The drawing under review shows one solid part. Ordinate dimensions are in mm from its lowest x, y, z. A direction names the side the tool comes from. Coordinates: 2 decimals unless noted, no trailing zeros. Loops run counter-clockwise (first coordinate to the right, second up) from the corner with the lowest first, then second, coordinate; pieces in that order, holes last. Notation, with made-up numbers: (2.5, 50) -> (58.5, 50) arc R27 ccw to (58.5, 69) -> close; hole circle Ø3 at (-39.5, 45.5). An arc over 180 degrees is marked (long way). Use a Markdown table: item, result.
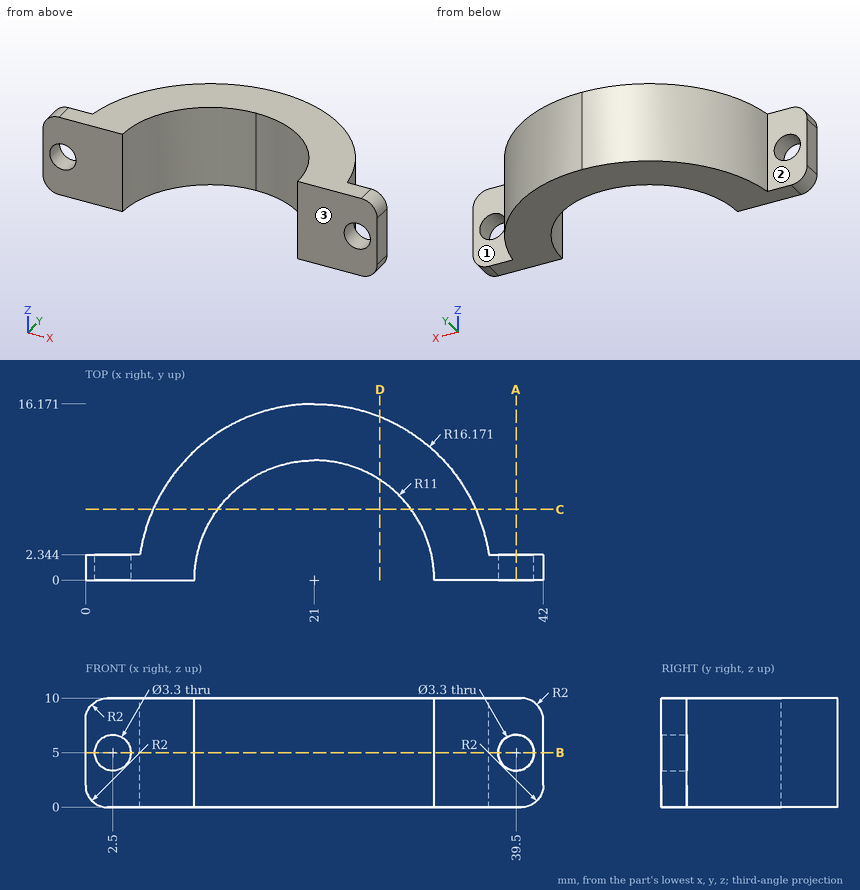
(1) Take a section at C-C on y = 6.5. Write out the cut boundary in (x, z), plus the area to 3 significant figures.
Found:
| item | result |
|---|---|
| outline | (6.19, 0) -> (12.13, 0) -> (12.13, 10) -> (6.19, 10) -> close; (29.87, 0) -> (35.81, 0) -> (35.81, 10) -> (29.87, 10) -> close |
| area | 119 mm^2 |
(2) For pin 1 Ø4 at (x, z) = (18, 2) entering from +Y; pin 2 Ø1.5 at (y, z) = (2.5, 1) entering from +X; pin 3 Ø1.5 at (x, z) = (38.5, 7) entering from +Y, all flat-tipped, find the tip position at first contact; note any pin that passes through.
Found:
| item | result |
|---|---|
| pin 1 | stops at y = 16.14 |
| pin 2 | stops at x = 41.98 |
| pin 3 | stops at y = 2.34 |
(3) For the marked faces 1, 2 and 3, list the 3-axis set-ups (+Z, -Z, +X, -X, +Y, -Y) from which the entire face can be reached by the end or side of a thin tool; tool diameter is ignored.
Found:
| item | result |
|---|---|
| face 1 | +Z, -Z, +X, +Y |
| face 2 | +Z, -Z, -X, +Y |
| face 3 | +Z, -Z, +X, -X, -Y |
(4) Take a section at D-D on x = 27. Write out the cut boundary in (y, z).
Found:
| item | result |
|---|---|
| outline | (9.22, 0) -> (15.02, 0) -> (15.02, 10) -> (9.22, 10) -> close |
(5) Take a section at B-B on z = 5. Write out the cut boundary in (x, y).
Found:
| item | result |
|---|---|
| outline | (0, 0) -> (0.85, 0) -> (0.85, 2.34) -> (0, 2.34) -> close; (4.15, 0) -> (10, 0) arc R11 cw to (32, 0) -> (37.85, 0) -> (37.85, 2.34) -> (37, 2.34) arc R16.17 ccw to (5, 2.34) -> (4.15, 2.34) -> close; (41.15, 0) -> (42, 0) -> (42, 2.34) -> (41.15, 2.34) -> close |
(6) Take a section at A-A on x = 39.5. Write out the cut boundary in (y, z), plus the area to 3 significant figures.
Found:
| item | result |
|---|---|
| outline | (0, 0) -> (2.34, 0) -> (2.34, 3.35) -> (0, 3.35) -> close; (0, 6.65) -> (2.34, 6.65) -> (2.34, 10) -> (0, 10) -> close |
| area | 15.7 mm^2 |
(7) For line 1 along Z through (x, y) = (39.5, 1.3); line 2 along X through (y, z) = (1.75, 5); line 3 along X through (y, z) = (0.9, 5), list the stretches that pass through material, from the lowest coordinate up.
Found:
| item | result |
|---|---|
| line 1 | z = 0 to 3.35, 6.65 to 10 |
| line 2 | x = 0 to 0.85, 4.15 to 10.14, 31.86 to 37.85, 41.15 to 42 |
| line 3 | x = 0 to 0.85, 4.15 to 10.04, 31.96 to 37.85, 41.15 to 42 |
